Part model, mm, in its own coordinate system. A direction names the side the tool comes from. Round coordinates to 2 decimals unless told otherwise and drop trailing zeros. Order: outer loops, then holes, each group sorted by start corner. A loop starts at its lowest first (then second) coordinate and runs counter-clockwise, first axis right, second up. Notation, with made-up numbers: (2, 66.25) -> (12, 66.25) arc R32 cw to (12, 104.25) -> close; hole circle Ø9 at (54.5, 9). An arc over 180 degrees is marked (long way). Return JSON: item names as keys, results as strings. Group by question number.
from build123d import *

# Parameters (mm, degrees)
BOSS_EXTRUDE1_DEPTH = 70
SKETCH2_R           = 7.5
CUT_EXTRUDE1_DEPTH  = 9
SKETCH3_R           = 7.5
CUT_EXTRUDE2_DEPTH  = 9
BOSS_EXTRUDE7_DEPTH = 9
BOSS_EXTRUDE8_DEPTH = 9
SKETCH8_W           = 32
SKETCH8_H           = 6
BOSS_EXTRUDE9_DEPTH = 46
SKETCH10_R          = 7.5
CUT_EXTRUDE3_DEPTH  = 46


with BuildPart() as part:
    # Sketch1 → Boss-Extrude1 (new body)
    with BuildSketch(Plane(origin=(0, 0, 0), x_dir=(1, 0, 0), z_dir=(0, 1, 0))):
        Polygon((0, 0), (120, 0), (120, -9), (85, -9), (85, -22.792607803), (76, -22.792607803), (76, -10.22587269), (44, -10.22587269), (44, -22.792607803), (35, -22.792607803), (35, -10.22587269), (0, -10.22587269), align=None)
    extrude(amount=BOSS_EXTRUDE1_DEPTH)

    # Sketch2 → Cut-Extrude1 (cut)
    with BuildSketch(Plane.XY.offset(9)):
        with Locations((102, 40)):
            Circle(SKETCH2_R)
    extrude(amount=-CUT_EXTRUDE1_DEPTH, mode=Mode.SUBTRACT)

    # Sketch3 → Cut-Extrude2 (cut)
    with BuildSketch(Plane.XY.offset(10.22587269)):
        with Locations((18, 40)):
            Circle(SKETCH3_R)
    extrude(amount=-CUT_EXTRUDE2_DEPTH, mode=Mode.SUBTRACT)

    # Sketch4 → Boss-Extrude7 (add)
    with BuildSketch(Plane(origin=(85, 0, 0), x_dir=(0, 0, -1), z_dir=(1, 0, 0))):
        Polygon((-56.792607803, 0), (-22.792607803, 0), (-22.792607803, 70), (-56.792607803, 6), align=None)
    extrude(amount=-BOSS_EXTRUDE7_DEPTH)

    # Sketch7 → Boss-Extrude8 (add)
    with BuildSketch(Plane.ZY.offset(-35)):
        Polygon((22.792607803, 0), (56.792607803, 0), (56.792607803, 6), (22.792607803, 70), align=None)
    extrude(amount=-BOSS_EXTRUDE8_DEPTH)

    # Sketch8 → Boss-Extrude9 (add)
    with BuildSketch(Plane.XY.offset(56.792607803)):
        with Locations((60, 3)):
            Rectangle(SKETCH8_W, SKETCH8_H)
    extrude(amount=-BOSS_EXTRUDE9_DEPTH)

    # Sketch10 → Cut-Extrude3 (cut)
    with BuildSketch(Plane.XY.offset(1.22587269)):
        with Locations((18, 40)):
            Circle(SKETCH10_R)
    extrude(amount=-CUT_EXTRUDE3_DEPTH, mode=Mode.SUBTRACT)


solid = part.part
(1) Saw through at C-C, the plane z = 6.5. List the corners of the cut face in (x, y).
(2) Saw through at A-A, the plane x = 102. List the corners of the cut face in (y, z).
(3) Pin check, flat tips, straight feed: P1, Ø10, axis at y = 54.5, z = 37, coming from the -X side; P2, Ø10.5, axis at x = 94.5, y = 52, coming from the +Z side; P3, Ø12, axis at y = 20, z = 48, coming from the +X side; P4, Ø14, axis at y = 38, z = 29.5, coming from the -X side. Stop position of each tip, or through.
(4) Saw through at D-D, the plane x = 80.5. List the corners of the cut face in (y, z), and give its area (3 significant figures).
(5) Mould opens along Y. For faces 1 (the flat face through (60, 3, 10.793)), 2 (the flat face through (60, 6, 34)), 3 (the cylindrical face through (100.37, 32.68, 4.56)) say: pulls with the +Y half, pulls with the -Y half, needs draft (parallel to the pull), parting line crosses it, or undercut.
(6) Tool access for faces 4 (the flat face through (120, 35, 4)), 5 (the flat face through (103, 27, 9)), 6 (the flat face through (35, 28, 28)): list every direction of +Z, -Z, +X, -X, +Y, -Y with a clear straight run to the whole face (end or side of a thin tool).
(7) Saw through at B-B, the plane y = 40. List the corners of the cut face in (x, z), and give its area (3 significant figures).
(8) Probe L1, parallel to Y at x = 18.5, z = 2; L2, parallel to X at y = 24, z = 36; L3, parallel to Z at x = 65, y = 4. List the from-to ranges inside material, lowest first. Write a range as [from, to].
Results are:
{
 "1": {"outline": "(0, 0) -> (120, 0) -> (120, 70) -> (0, 70) -> close; hole circle Ø15 at (18, 40); hole circle Ø15 at (102, 40)"},
 "2": {"outline": "(0, 0) -> (32.5, 0) -> (32.5, 9) -> (0, 9) -> close; (47.5, 0) -> (70, 0) -> (70, 9) -> (47.5, 9) -> close"},
 "3": {"P1": "passes through", "P2": "stops at z = 9", "P3": "stops at x = 85", "P4": "stops at x = 35"},
 "4": {"outline": "(0, 0) -> (70, 0) -> (70, 22.79) -> (6, 56.79) -> (0, 56.79) -> close", "area": "2,890 mm^2"},
 "5": {"face 1": "needs draft", "face 2": "pulls with the +Y half", "face 3": "undercut"},
 "6": {"face 4": "+Z, -Z, +X, +Y, -Y", "face 5": "+Z, +X, +Y, -Y", "face 6": "+Z, -X, +Y, -Y"},
 "7": {"outline": "(0, 0) -> (10.5, 0) -> (10.5, 10.23) -> (0, 10.23) -> close; (25.5, 0) -> (94.5, 0) -> (94.5, 9) -> (85, 9) -> (85, 38.73) -> (76, 38.73) -> (76, 10.23) -> (44, 10.23) -> (44, 38.73) -> (35, 38.73) -> (35, 10.23) -> (25.5, 10.23) -> close; (109.5, 0) -> (120, 0) -> (120, 9) -> (109.5, 9) -> close", "area": "1,410 mm^2"},
 "8": {"L1": "y = [0, 32.52], [47.48, 70]", "L2": "x = [35, 44], [76, 85]", "L3": "z = [0, 10.23], [10.79, 56.79]"}
}
